CAD build for the part. Positions are in the model's coordinates, mm. Round coordinates to 2 decimals unless told otherwise and drop trailing zeros. Order: outer loops, then holes, each group sorted by start corner. A loop starts at its lowest first (then second) coordinate and runs counter-clockwise, first axis right, second up.
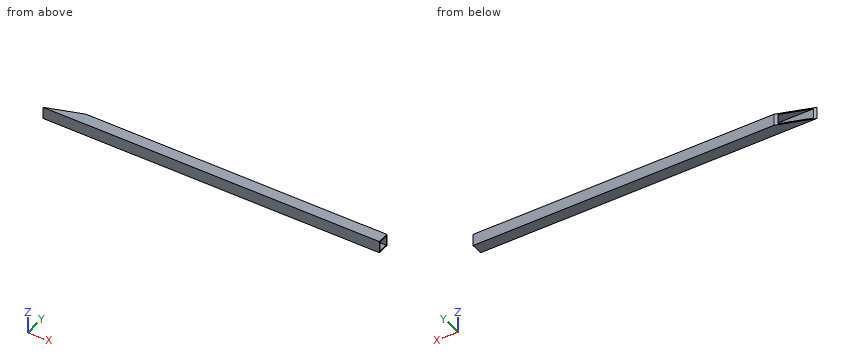
```python
from build123d import *

# Parameters (mm, degrees)
SKETCH_W     = 31.75
SKETCH_H     = 31.75
SKETCH_W_2   = 26.2128
SKETCH_H_2   = 26.2128
PAD_DEPTH    = 909.258
POCKET_DEPTH = 31.75


with BuildPart() as part:
    # Sketch → Pad (new body)
    with BuildSketch(Plane.YZ):
        Rectangle(SKETCH_W, SKETCH_H)
        Rectangle(SKETCH_W_2, SKETCH_H_2, mode=Mode.SUBTRACT)
    extrude(amount=-PAD_DEPTH)

    # Sketch001 → Pocket (cut)
    with BuildSketch(Plane(origin=(0, 0, 15.875), x_dir=(0, -1, 0), z_dir=(0, 0, 1))):
        Polygon((15.875, -909.258), (-15.875, -909.258), (-15.875, -814.007729), align=None)
    extrude(amount=-POCKET_DEPTH, mode=Mode.SUBTRACT)


solid = part.part
```
1. Cut at A-A, the plane z = 0. Write the cut outline in (x, y) (3 decimals), and give its area (3 significant figures).
2. Cut at C-C, the plane y = 1. Write the cut outline in (x, z) (3 decimals), and give its area (3 significant figures).
3. Cut at B-B, the plane x = -454. Write the cut outline in (y, z) (3 decimals), and give its area (3 significant figures).
4. Drill centre line: line 1 (Y direction, x = -193.5, z = 3) (3 decimals). Where is it in solid material? Low to high.
Outcome:
1. outline: (-909.258, -15.875) - (0, -15.875) - (0, -13.106) - (-900.952, -13.106) - close; (-822.314, 13.106) - (0, 13.106) - (0, 15.875) - (-814.008, 15.875) - close
1. area: 4,770 mm2
2. outline: (-858.633, -15.875) - (0, -15.875) - (0, -13.106) - (-858.633, -13.106) - close; (-858.633, 13.106) - (0, 13.106) - (0, 15.875) - (-858.633, 15.875) - close
2. area: 4,750 mm2
3. outline: (-15.875, -15.875) - (15.875, -15.875) - (15.875, 15.875) - (-15.875, 15.875) - close; hole (-13.106, -13.106) - (13.106, -13.106) - (13.106, 13.106) - (-13.106, 13.106) - close
3. area: 321 mm2
4. line 1: y = -15.875 to -13.106, 13.106 to 15.875
